Can you work these out from the model? Positions are in its coordinate system, mm. Face numbers are marked on the shaded views. A direction names the side the tool comes from. Round coordinates to 2 decimals unless told otherwise and drop trailing zeros. Loops run counter-clockwise (first coordinate to the right, second up) from the corner with the lowest first, then second, coordinate; pieces in that order, holes last. Notation, with made-up numbers: (-35.5, 69) - (2.5, 69) arc R14 cw to (2.5, 81) - close; hole circle Ø4 at (87, -35.75). An arc over 180 degrees is marked (long way). Answer as CSV lines item,"result".
```python
from build123d import *

# Parameters (mm, degrees)
F0_W      = 711.2
F0_H      = 558.8
F1_DEPTH  = 19.05
F2_W      = 622.3
F2_H      = 19.05
F3_DEPTH  = 88.9
F4_W      = 19.05
F4_H      = 469.9
F5_DEPTH  = 88.9
F6_W      = 88.9
F6_H      = 19.05
F7_DEPTH  = 457.2
F9_W      = 546.1
F9_H      = 19.05
F10_DEPTH = 76.2
F11_W     = 19.05
F11_H     = 431.8
F12_DEPTH = 44.45
F14_DEPTH = 19.05
F16_DEPTH = 19.05


with BuildPart() as f1:
    # F0 (on Top) → F1 (new body)
    with BuildSketch(Plane.XY):
        Rectangle(F0_W, F0_H)
    extrude(amount=-F1_DEPTH)

    # F2 (on face) → F3 (join)
    with BuildSketch(Plane(origin=(0, 0, -19.05), x_dir=(1, 0, 0), z_dir=(0, 0, -1))):
        with Locations((0, 244.475)):
            Rectangle(F2_W, F2_H)
        with Locations((0, -244.475)):
            Rectangle(F2_W, F2_H)
    extrude(amount=F3_DEPTH)

    # F4 (on face) → F5 (join)
    with BuildSketch(Plane(origin=(0, 0, -19.05), x_dir=(1, 0, 0), z_dir=(0, 0, -1))):
        with Locations((-301.625, 0)):
            Rectangle(F4_W, F4_H)
        with Locations((301.625, 0)):
            Rectangle(F4_W, F4_H)
    extrude(amount=F5_DEPTH)

    # F6 (on face) → F7 (join)
    with BuildSketch(Plane(origin=(0, 0, -19.05), x_dir=(1, 0, 0), z_dir=(0, 0, -1))):
        Polygon((-273.05, 234.95), (-292.1, 234.95), (-292.1, 146.05), (-273.05, 146.05), (-273.05, 215.9), align=None)
        with Locations((-228.6, 225.425)):
            Rectangle(F6_W, F6_H)
        Polygon((292.1, 184.15), (292.1, 234.95), (273.05, 234.95), (273.05, 215.9), (273.05, 146.05), (292.1, 146.05), align=None)
        with Locations((228.6, 225.425)):
            Rectangle(F6_W, F6_H)
        Polygon((273.05, -234.95), (292.1, -234.95), (292.1, -184.15), (292.1, -146.05), (273.05, -146.05), (273.05, -215.9), align=None)
        with Locations((228.6, -225.425)):
            Rectangle(F6_W, F6_H)
        Polygon((-292.1, -146.05), (-292.1, -234.95), (-273.05, -234.95), (-273.05, -215.9), (-273.05, -146.05), align=None)
        with Locations((-228.6, -225.425)):
            Rectangle(F6_W, F6_H)
    extrude(amount=F7_DEPTH)

    # F9 (on face) → F10 (join)
    with BuildSketch(Plane(origin=(0, 0, -349.25), x_dir=(1, 0, 0), z_dir=(0, 0, -1))):
        with Locations((0, -206.375)):
            Rectangle(F9_W, F9_H)
        with Locations((0, 206.375)):
            Rectangle(F9_W, F9_H)
    extrude(amount=F10_DEPTH)

    # F11 (on face) → F12 (join)
    with BuildSketch(Plane(origin=(0, 0, -349.25), x_dir=(1, 0, 0), z_dir=(0, 0, -1))):
        Polygon((254, -215.9), (273.05, -215.9), (273.05, 215.9), (254, 215.9), (254, 0), align=None)
        with Locations((-263.525, 0)):
            Rectangle(F11_W, F11_H)
    extrude(amount=-F12_DEPTH)

    # F13 (on face) → F14 (join)
    with BuildSketch(Plane(origin=(273.05, 0, 0), x_dir=(0, -1, 0), z_dir=(-1, 0, 0))):
        Polygon((-144.0579510314, -19.05), (-215.9, -90.8920489686), (-215.9, -153.753841816), (-81.196158184, -19.05), align=None)
        Polygon((215.9, -153.753841816), (215.9, -90.8920489686), (144.0579510314, -19.05), (81.196158184, -19.05), align=None)
    extrude(amount=F14_DEPTH)

    # F15 (on face) → F16 (join)
    with BuildSketch(Plane.YZ.offset(-273.05)):
        Polygon((-144.0579510314, -19.05), (-215.9, -90.8920489686), (-215.9, -153.753841816), (-81.196158184, -19.05), align=None)
        Polygon((144.0579510314, -19.05), (81.196158184, -19.05), (215.9, -153.753841816), (215.9, -90.8920489686), align=None)
    extrude(amount=F16_DEPTH)


solid = f1.part
```
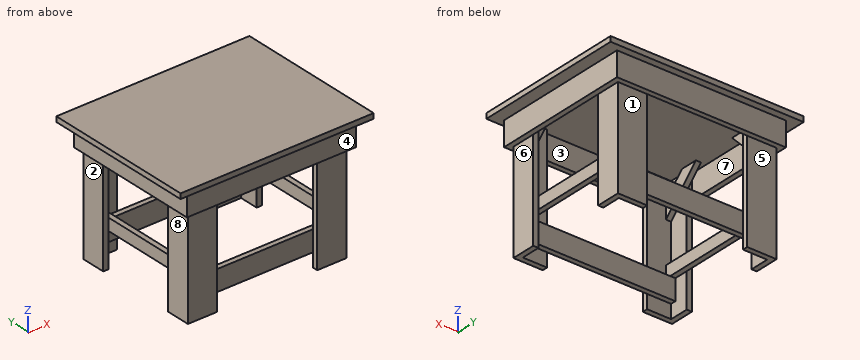
Q1. Imagine slicing it at A-A (y = 62.5). Write out the boundary of the cut face in (x, z), then the cut area to 3 significant figures.
Checks:
outline,"(-355.6, -19.05) - (-311.15, -19.05) - (-311.15, -107.95) - (-292.1, -107.95) - (-292.1, -19.05) - (292.1, -19.05) - (292.1, -107.95) - (311.15, -107.95) - (311.15, -19.05) - (355.6, -19.05) - (355.6, 0) - (-355.6, 0) - close; (-273.05, -349.25) - (-254, -349.25) - (-254, -304.8) - (-273.05, -304.8) - close; (254, -349.25) - (273.05, -349.25) - (273.05, -304.8) - (254, -304.8) - close"
area,"18,600 mm²"
Q2. On a 3-axis mill with a long thin cutter (end or side, diameter ignored), from which of +Z, -Z, +X, -X, +Y, -Y can I reach the whole of each face in a straight line? I mean the marked faces 4, 5, 6, 7 and 8. Say none if no direction works.
Checks:
face 4,"-Z, +X, -X, -Y"
face 5,"-Z, +X, -X, +Y"
face 6,"-Z, +X, +Y, -Y"
face 7,"-Z"
face 8,"-Z, -X, +Y, -Y"
Q3. I'm going to push flat-ended pins straight in: pin 1 Ø2 at (x, y) = (-131, -123) entering from -Z; pin 2 Ø21 at (y, z) = (193.5, -381.5) entering from +X; pin 3 Ø2 at (x, z) = (-93.5, -353) entering from +Y; pin 4 Ø10 at (y, z) = (139.5, -233.5) entering from +X. Where does each tip first touch, or does it pass through?
Checks:
pin 1,"z = -19.05"
pin 2,"x = 292.1"
pin 3,"y = 215.9"
pin 4,"through"
Q4. Imagine slicing it at C-C (z = -373.5). Write out the boundary of the cut face in (x, y).
Checks:
outline,"(-292.1, -234.95) - (-184.15, -234.95) - (-184.15, -215.9) - (184.15, -215.9) - (184.15, -234.95) - (292.1, -234.95) - (292.1, -146.05) - (273.05, -146.05) - (273.05, -196.85) - (-273.05, -196.85) - (-273.05, -146.05) - (-292.1, -146.05) - close; (-292.1, 146.05) - (-273.05, 146.05) - (-273.05, 196.85) - (273.05, 196.85) - (273.05, 146.05) - (292.1, 146.05) - (292.1, 234.95) - (184.15, 234.95) - (184.15, 215.9) - (-184.15, 215.9) - (-184.15, 234.95) - (-292.1, 234.95) - close"
Q5. If I drill on line 1 along X through (y, z) = (125.5, -26); line 2 along Y through (x, z) = (-112, -28); line 3 along Y through (x, z) = (92, -392), over which ranges is the centre line in solid material (lowest first)? Write a range as [from, to].
Checks:
line 1,"[-311.15, -292.1], [-273.05, -254], [254, 273.05], [292.1, 311.15]"
line 2,"[-254, -234.95], [234.95, 254]"
line 3,"[-215.9, -196.85], [196.85, 215.9]"
Q6. Imagine slicing it at B-B (x = 88). Write out the boundary of the cut face in (y, z).
Checks:
outline,"(-279.4, -19.05) - (-254, -19.05) - (-254, -107.95) - (-234.95, -107.95) - (-234.95, -19.05) - (234.95, -19.05) - (234.95, -107.95) - (254, -107.95) - (254, -19.05) - (279.4, -19.05) - (279.4, 0) - (-279.4, 0) - close; (-215.9, -425.45) - (-196.85, -425.45) - (-196.85, -349.25) - (-215.9, -349.25) - close; (196.85, -425.45) - (215.9, -425.45) - (215.9, -349.25) - (196.85, -349.25) - close"
Q7. Imagine slicing it at D-D (z = -179.5). Write out the boundary of the cut face in (x, y), then the cut area to 3 significant figures.
Checks:
outline,"(-292.1, -234.95) - (-184.15, -234.95) - (-184.15, -215.9) - (-273.05, -215.9) - (-273.05, -146.05) - (-292.1, -146.05) - close; (-292.1, 146.05) - (-273.05, 146.05) - (-273.05, 215.9) - (-184.15, 215.9) - (-184.15, 234.95) - (-292.1, 234.95) - close; (184.15, -234.95) - (292.1, -234.95) - (292.1, -146.05) - (273.05, -146.05) - (273.05, -215.9) - (184.15, -215.9) - close; (184.15, 215.9) - (273.05, 215.9) - (273.05, 146.05) - (292.1, 146.05) - (292.1, 234.95) - (184.15, 234.95) - close"
area,"13,500 mm²"
Q8. We'd pull the mould along X, two halves only. Please class the marked faces 1, 2 and 3: pulls with the +X half, pulls with the -X half, needs draft (parallel to the pull), parting line crosses it, or undercut.
Checks:
face 1,"needs draft"
face 2,"pulls with the -X half"
face 3,"undercut"
